Design review of the part built by this model. Coordinates are the model's own, in mm. A direction names the side the tool comes from. Give positions to 0.01 mm unless a question says otherwise; leave off trailing zeros. Write each loop counter-clockwise with the first axis right and the second up, starting at its lowest first coordinate (ties: lowest second). Pieces come first, ordered by that corner, then holes. Notation, with made-up numbers: (74, -1) -> (92, -1) arc R24 ccw to (92, 38) -> close; hole circle Ø8 at (-18, -1.75). An arc over 180 degrees is marked (long way). Return JSON: item names as keys, results as strings. Group by question number.
from build123d import *

# Parameters (mm, degrees)
SKETCH_1_W                   = 120
SKETCH_1_H                   = 20
EXTRUDE_1_DEPTH              = 8
SKETCH_2_W                   = 50
SKETCH_2_H                   = 14
CUT_EXTRUDE_1_DEPTH          = 122.918005233
HOLE_WIZARD_M4_1_D           = 4.8
HOLE_WIZARD_M4_1_CBORE_D     = 8
HOLE_WIZARD_M4_1_CBORE_DEPTH = 4


with BuildPart() as part:
    # 草图1 → 凸台-拉伸1 (new body)
    with BuildSketch(Plane.XY):
        with Locations((60, 10)):
            Rectangle(SKETCH_1_W, SKETCH_1_H)
    extrude(amount=EXTRUDE_1_DEPTH)

    # 草图2 → 切除-拉伸1 (cut, through all)
    with BuildSketch(Plane.XY.offset(8)):
        with Locations((60, 13)):
            Rectangle(SKETCH_2_W, SKETCH_2_H)
    extrude(amount=-CUT_EXTRUDE_1_DEPTH, mode=Mode.SUBTRACT)

    # M4 六角凹头螺钉的柱形沉头孔1 (through all)
    with Locations(Plane.XY.offset(8)):
        with Locations((12, 10), (27, 10), (93, 10), (108, 10)):
            CounterBoreHole(HOLE_WIZARD_M4_1_D / 2, HOLE_WIZARD_M4_1_CBORE_D / 2, HOLE_WIZARD_M4_1_CBORE_DEPTH)


solid = part.part
Q1. Take a section at D-D, the plane y = 10. Count the separate pieces of the cut face and the enclosed holes in it, plus the area to 3 significant figures.
Q2. Tool access review of faces 1 (the face through (35, 13, 4)), 2 (the face through (24.71, 10.72, 1.97)), 3 (the face through (23, 10, 6)): name each direction out of +Z, -Z, +X, -X, +Y, -Y from which nothing blocks a thin tool from reaching the whole face with its end or side.
Q3. Take a section at B-B, the plane y = 16.75. Give the boundary of the cut face in (x, z), plus the area to 3 significant figures.
Q4. Take a section at A-A, the plane x = 27. Give the boundary of the cut face in (y, z), plus the area to 3 significant figures.
Q5. Insertion check: pin 1 (2.5 mm diameter, centred on x = 109.5, y = 9.5, fed in from +Z); pin 2 (3 mm diameter, centred on x = 93, y = 10, fed in from +Z). Each pin has a flat end and moves straight along its axis. Give the tip position at first contact, or say it passes through.
Q6. Take a section at C-C, the plane z = 5. Give the boundary of the cut face in (x, y).
Q7. For L1, parallel to X at y = 16, z = 3.25; L2, parallel to Y at x = 108, z = 5.15; L3, parallel to Y at x = 27, z = 1.6, list the stretches that pass through material, from the lowest coordinate up. Write a range as from..to.
Q8. Mouldability with a two-part tool opening along X and no side actions: class faces 4 (the face through (85, 13, 4)), 5 (the face through (90.783, 9.081, 1.972)), 6 (the face through (120, 10, 4)), 7 (the face through (59, 0, 4)) as +X half, -X half, draft (parallel to the pull), parting line (faces both ways), or undercut.
Final values:
{
 "1": {"separate pieces": "6", "enclosed holes": "0", "area": "355 mm²"},
 "2": {"face 1": "+Z, -Z, +Y", "face 2": "+Z, -Z", "face 3": "+Z"},
 "3": {"outline": "(0, 0) -> (35, 0) -> (35, 8) -> (0, 8) -> close; (85, 0) -> (120, 0) -> (120, 8) -> (85, 8) -> close", "area": "560 mm²"},
 "4": {"outline": "(0, 0) -> (7.6, 0) -> (7.6, 4) -> (6, 4) -> (6, 8) -> (0, 8) -> close; (12.4, 0) -> (20, 0) -> (20, 8) -> (14, 8) -> (14, 4) -> (12.4, 4) -> close", "area": "109 mm²"},
 "5": {"pin 1": "stops at z = 4", "pin 2": "passes through"},
 "6": {"outline": "(0, 0) -> (120, 0) -> (120, 20) -> (85, 20) -> (85, 6) -> (35, 6) -> (35, 20) -> (0, 20) -> close; hole circle Ø8 at (12, 10); hole circle Ø8 at (27, 10); hole circle Ø8 at (93, 10); hole circle Ø8 at (108, 10)"},
 "7": {"L1": "x = 0..35, 85..120", "L2": "y = 0..6, 14..20", "L3": "y = 0..7.6, 12.4..20"},
 "8": {"face 4": "undercut", "face 5": "undercut", "face 6": "+X half", "face 7": "draft"}
}
